```python
from build123d import *

# Parameters (mm, degrees)
SKETCH_1_W             = 35
SKETCH_1_H             = 70
SKETCH_1_R             = 2.6
EXTRUDE_528_DEPTH      = 3
SKETCH_2_R             = 2.1
CUT_EXTRUDE_M4_DEPTH   = 3
SKETCH_3_R             = 2.6
EXTRUDE_990_DEPTH      = 3
SKETCH_4_R             = 2.1
CUT_EXTRUDE_1335_DEPTH = 4
SKETCH_5_W             = 49
SKETCH_5_H             = 70
EXTRA_DEPTH            = 3
SKETCH_6_R             = 2.1
CUT_EXTRUDE_2079_DEPTH = 10
SKETCH_7_R             = 2.1
ETRA_DEPTH             = 10
SKETCH_10_R            = 1.6
SKETCH_10_R_2          = 3.5
CUT_EXTRUDE_3705_DEPTH = 4
FILLET_5_0_R           = 5
SKETCH_12_R            = 2.1
EXTRUDE_1_DEPTH        = 3
SKETCH_13_R            = 1.5
CUT_EXTRUDE_1_DEPTH    = 4
SKETCH_14_R            = 1.5
EXTRUDE_2_DEPTH        = 3
SKETCH_15_R            = 2.5
CUT_EXTRUDE_2_DEPTH    = 4
SKETCH_16_R            = 2.6
EXTRUDE_3_DEPTH        = 3
SKETCH_18_R            = 2.5
CUT_EXTRUDE_3_DEPTH    = 3
SKETCH_19_R            = 2.180798689
SKETCH_19_R_2          = 1.661770768
EXTRUDE_4_DEPTH        = 3
SKETCH_20_R            = 2.5
CUT_EXTRUDE_4_DEPTH    = 4
SKETCH_21_R            = 1.5
SKETCH_21_R_2          = 2.5
SKETCH_21_R_3          = 2.1
EXTRUDE_5_DEPTH        = 3
SKETCH_22_R            = 1.5
CUT_EXTRUDE_5_DEPTH    = 4
SKETCH_23_R            = 1.5
EXTRUDE_6_DEPTH        = 3
SKETCH_24_R            = 1.2
CUT_EXTRUDE_8_DEPTH    = 4
SKETCH_26_R            = 1.5
CUT_EXTRUDE_10_DEPTH   = 4
SKETCH_27_R            = 1.2
SKETCH_27_R_2          = 1.228912634
EXTRUDE_7_DEPTH        = 3
SKETCH_28_R            = 2.5
EXTRUDE_8_DEPTH        = 3
SKETCH_29_R            = 1.2
CUT_EXTRUDE_11_DEPTH   = 4
SKETCH_30_R            = 1.5
EXTRUDE_9_DEPTH        = 3
SKETCH_31_R            = 2.5
CUT_EXTRUDE_12_DEPTH   = 4
SKETCH_32_R            = 2.622023652
SKETCH_32_R_2          = 2.1
EXTRUDE_10_DEPTH       = 3
SKETCH_34_R            = 2.5
EXTRUDE_11_DEPTH       = 3
SKETCH_35_R            = 1.2
CUT_EXTRUDE_13_DEPTH   = 4
SKETCH_37_R            = 1.6
SKETCH_37_R_2          = 2.6
CUT_EXTRUDE_14_DEPTH   = 4


with BuildPart() as part:
    # 草图1 → Extrude 528 (new body)
    with BuildSketch(Plane(origin=(0, 0, 0), x_dir=(1, 0, 0), z_dir=(0, 1, 0))):
        Rectangle(SKETCH_1_W, SKETCH_1_H)
        with Locations((-7.5, 22.5)):
            Circle(SKETCH_1_R, mode=Mode.SUBTRACT)
        with Locations((-7.5, 0)):
            Circle(SKETCH_1_R, mode=Mode.SUBTRACT)
        with Locations((-7.5, -22.5)):
            Circle(SKETCH_1_R, mode=Mode.SUBTRACT)
        with Locations((-7.5, 10)):
            Circle(SKETCH_1_R, mode=Mode.SUBTRACT)
        with Locations((-7.5, -10)):
            Circle(SKETCH_1_R, mode=Mode.SUBTRACT)
    extrude(amount=EXTRUDE_528_DEPTH)

    # 草图2 → M4铝柱 (cut)
    with BuildSketch(Plane(origin=(0, 3, 0), x_dir=(1, 0, 0), z_dir=(0, 1, 0))):
        with Locations((10, 0)):
            Circle(SKETCH_2_R)
    extrude(amount=-CUT_EXTRUDE_M4_DEPTH, mode=Mode.SUBTRACT)

    # 草图3 → Extrude 990 (add, through all)
    with BuildSketch(Plane(origin=(0, 3, 0), x_dir=(1, 0, 0), z_dir=(0, 1, 0))):
        with Locations((-7.5, -10)):
            Circle(SKETCH_3_R)
        with Locations((-7.5, 10)):
            Circle(SKETCH_3_R)
    extrude(amount=-EXTRUDE_990_DEPTH)

    # 草图4 → Cut-Extrude 1335 (cut, through all)
    with BuildSketch(Plane(origin=(0, 3, 0), x_dir=(1, 0, 0), z_dir=(0, 1, 0))):
        with Locations((10, 22.5)):
            Circle(SKETCH_4_R)
        with Locations((10, -22.5)):
            Circle(SKETCH_4_R)
    extrude(amount=-CUT_EXTRUDE_1335_DEPTH, mode=Mode.SUBTRACT)

    # 草图5 → EXTRA (add, through all)
    with BuildSketch(Plane(origin=(0, 3, 0), x_dir=(1, 0, 0), z_dir=(0, 1, 0))):
        with Locations((-42, 0)):
            Rectangle(SKETCH_5_W, SKETCH_5_H)
    extrude(amount=-EXTRA_DEPTH)

    # 草图6 → Cut-Extrude 2079 (cut)
    with BuildSketch(Plane(origin=(0, 3, 0), x_dir=(1, 0, 0), z_dir=(0, 1, 0))):
        with Locations((-44.5, 0)):
            Circle(SKETCH_6_R)
        with Locations((-36.5, 0)):
            Circle(SKETCH_6_R)
    extrude(amount=-CUT_EXTRUDE_2079_DEPTH, mode=Mode.SUBTRACT)

    # 草图7 → ETRA铝柱 (cut)
    with BuildSketch(Plane(origin=(0, 3, 0), x_dir=(1, 0, 0), z_dir=(0, 1, 0))):
        with Locations((-56.5, 17.5)):
            Circle(SKETCH_7_R)
        with Locations((-56.5, -17.5)):
            Circle(SKETCH_7_R)
    extrude(amount=-ETRA_DEPTH, mode=Mode.SUBTRACT)

    # 草图10 → Cut-Extrude 3705 (cut, through all)
    with BuildSketch(Plane.XZ):
        with Locations((-43.5, -21.25)):
            Circle(SKETCH_10_R)
        with Locations((-21.5, -31.75)):
            Circle(SKETCH_10_R)
        with Locations((-43.5, -31.75)):
            Circle(SKETCH_10_R)
        with Locations((-43.5, 21.25)):
            Circle(SKETCH_10_R)
        with Locations((-21.5, 31.75)):
            Circle(SKETCH_10_R)
        with Locations((-43.5, 31.75)):
            Circle(SKETCH_10_R)
        with Locations((-21.5, 21.25)):
            Circle(SKETCH_10_R_2)
        with Locations((-21.5, -21.25)):
            Circle(SKETCH_10_R_2)
    extrude(amount=-CUT_EXTRUDE_3705_DEPTH, mode=Mode.SUBTRACT)

    # 圆角5.0
    fillet_5_0_edges = [part.edges().sort_by_distance(p)[0] for p in [
        (-66.5, 1.5, 35),
        (-66.5, 1.5, -35),
        (17.5, 1.5, 35),
        (17.5, 1.5, -35),
    ]]
    fillet(fillet_5_0_edges, radius=FILLET_5_0_R)

    # 草图12 → 凸台-拉伸1 (add)
    with BuildSketch(Plane(origin=(0, 3, 0), x_dir=(1, 0, 0), z_dir=(0, 1, 0))):
        with Locations((-36.5, 0)):
            Circle(SKETCH_12_R)
        with Locations((-44.5, 0)):
            Circle(SKETCH_12_R)
    extrude(amount=-EXTRUDE_1_DEPTH)

    # 草图13 → 切除-拉伸1 (cut, through all)
    with BuildSketch(Plane(origin=(0, 3, 0), x_dir=(1, 0, 0), z_dir=(0, 1, 0))):
        with Locations((-52.499999555, 1.426e-06)):
            Circle(SKETCH_13_R)
        with Locations((-28.499999555, 1.44e-06)):
            Circle(SKETCH_13_R)
    extrude(amount=-CUT_EXTRUDE_1_DEPTH, mode=Mode.SUBTRACT)

    # 草图14 → 凸台-拉伸2 (add)
    with BuildSketch(Plane(origin=(0, 3, 0), x_dir=(1, 0, 0), z_dir=(0, 1, 0))):
        with Locations((-28.499999555, 1.44e-06)):
            Circle(SKETCH_14_R)
    extrude(amount=-EXTRUDE_2_DEPTH)

    # 草图15 → 切除-拉伸2 (cut, through all)
    with BuildSketch(Plane(origin=(0, 3, 0), x_dir=(1, 0, 0), z_dir=(0, 1, 0))):
        with Locations((-23.393651392, 12.166497951)):
            Circle(SKETCH_15_R)
        with Locations((-23.393651594, -11.919830539)):
            Circle(SKETCH_15_R)
    extrude(amount=-CUT_EXTRUDE_2_DEPTH, mode=Mode.SUBTRACT)

    # 草图16 → 凸台-拉伸3 (add)
    with BuildSketch(Plane(origin=(0, 3, 0), x_dir=(1, 0, 0), z_dir=(0, 1, 0))):
        with Locations((-7.5, 22.5)):
            Circle(SKETCH_16_R)
        with Locations((-7.5, 0)):
            Circle(SKETCH_16_R)
        with Locations((-7.5, -22.5)):
            Circle(SKETCH_16_R)
    extrude(amount=-EXTRUDE_3_DEPTH)

    # 草图18 → 切除-拉伸3 (cut)
    with BuildSketch(Plane.XZ):
        with Locations((-3.558761246, 0)):
            Circle(SKETCH_18_R)
        with Locations((-3.558761246, 22.202338419)):
            Circle(SKETCH_18_R)
        with Locations((-3.558761246, -23.518793957)):
            Circle(SKETCH_18_R)
    extrude(amount=-CUT_EXTRUDE_3_DEPTH, mode=Mode.SUBTRACT)

    # 草图19 → 凸台-拉伸4 (add)
    with BuildSketch(Plane.XZ):
        with Locations((-43.5, 21.25)):
            Circle(SKETCH_19_R)
        with Locations((-43.5, 31.75)):
            Circle(SKETCH_19_R_2)
    extrude(amount=-EXTRUDE_4_DEPTH)

    # 草图20 → 切除-拉伸4 (cut, through all)
    with BuildSketch(Plane(origin=(0, 3, 0), x_dir=(1, 0, 0), z_dir=(0, 1, 0))):
        with Locations((-40.5, 1.551947464)):
            Circle(SKETCH_20_R)
        with Locations((-40.5, -18.448052536)):
            Circle(SKETCH_20_R)
    extrude(amount=-CUT_EXTRUDE_4_DEPTH, mode=Mode.SUBTRACT)

    # 草图21 → 凸台-拉伸5 (add)
    with BuildSketch(Plane(origin=(0, 3, 0), x_dir=(1, 0, 0), z_dir=(0, 1, 0))):
        with Locations((-52.499999555, 1.426e-06)):
            Circle(SKETCH_21_R)
        with Locations((-40.5, 1.551947464)):
            Circle(SKETCH_21_R_2)
        with Locations((-3.558761246, 0)):
            Circle(SKETCH_21_R_2)
        with Locations((10, 0)):
            Circle(SKETCH_21_R_3)
    extrude(amount=-EXTRUDE_5_DEPTH)

    # 草图22 → 切除-拉伸5 (cut, through all)
    with BuildSketch(Plane(origin=(0, 3, 0), x_dir=(1, 0, 0), z_dir=(0, 1, 0))):
        with Locations((-52.5, 0)):
            Circle(SKETCH_22_R)
        with Locations((-28.5, 0)):
            Circle(SKETCH_22_R)
    extrude(amount=-CUT_EXTRUDE_5_DEPTH, mode=Mode.SUBTRACT)

    # 草图23 → 凸台-拉伸6 (add)
    with BuildSketch(Plane(origin=(0, 3, 0), x_dir=(1, 0, 0), z_dir=(0, 1, 0))):
        with Locations((-52.5, 0)):
            Circle(SKETCH_23_R)
        with Locations((-28.5, 0)):
            Circle(SKETCH_23_R)
    extrude(amount=-EXTRUDE_6_DEPTH)

    # 草图24 → 切除-拉伸8 (cut, through all)
    with BuildSketch(Plane(origin=(0, 3, 0), x_dir=(1, 0, 0), z_dir=(0, 1, 0))):
        with Locations((-45.5, -0.064794531)):
            Circle(SKETCH_24_R)
        with Locations((-25.5, -0.064794531)):
            Circle(SKETCH_24_R)
    extrude(amount=-CUT_EXTRUDE_8_DEPTH, mode=Mode.SUBTRACT)

    # 草图26 → 切除-拉伸10 (cut, through all)
    with BuildSketch(Plane.XZ):
        with Locations((-52.5, 0)):
            Circle(SKETCH_26_R)
        with Locations((-28.5, 0)):
            Circle(SKETCH_26_R)
    extrude(amount=-CUT_EXTRUDE_10_DEPTH, mode=Mode.SUBTRACT)

    # 草图27 → 凸台-拉伸7 (add)
    with BuildSketch(Plane(origin=(0, 0, 0), x_dir=(-1, 0, 0), z_dir=(0, -1, 0))):
        with Locations((25.5, -0.064794531)):
            Circle(SKETCH_27_R)
        with Locations((45.5, -0.064794531)):
            Circle(SKETCH_27_R_2)
    extrude(amount=-EXTRUDE_7_DEPTH)

    # 草图28 → 凸台-拉伸8 (add)
    with BuildSketch(Plane(origin=(0, 3, 0), x_dir=(1, 0, 0), z_dir=(0, 1, 0))):
        with Locations((-3.558761246, -22.202338419)):
            Circle(SKETCH_28_R)
        with Locations((-3.558761246, 23.518793957)):
            Circle(SKETCH_28_R)
    extrude(amount=-EXTRUDE_8_DEPTH)

    # 草图29 → 切除-拉伸11 (cut, through all)
    with BuildSketch(Plane(origin=(0, 3, 0), x_dir=(1, 0, 0), z_dir=(0, 1, 0))):
        with Locations((-25.5, -0.064794531)):
            Circle(SKETCH_29_R)
        with Locations((-45.5, -0.064794531)):
            Circle(SKETCH_29_R)
    extrude(amount=-CUT_EXTRUDE_11_DEPTH, mode=Mode.SUBTRACT)

    # 草图30 → 凸台-拉伸9 (add)
    with BuildSketch(Plane(origin=(0, 3, 0), x_dir=(1, 0, 0), z_dir=(0, 1, 0))):
        with Locations((-28.5, 0)):
            Circle(SKETCH_30_R)
        with Locations((-52.5, 0)):
            Circle(SKETCH_30_R)
    extrude(amount=-EXTRUDE_9_DEPTH)

    # 草图31 → 切除-拉伸12 (cut, through all)
    with BuildSketch(Plane.XZ):
        with Locations((-5, 25.879055361)):
            Circle(SKETCH_31_R)
        with Locations((-5, -25.879055361)):
            Circle(SKETCH_31_R)
    extrude(amount=-CUT_EXTRUDE_12_DEPTH, mode=Mode.SUBTRACT)

    # 草图32 → 凸台-拉伸10 (add)
    with BuildSketch(Plane(origin=(0, 3, 0), x_dir=(1, 0, 0), z_dir=(0, 1, 0))):
        with Locations((10, -22.5)):
            Circle(SKETCH_32_R)
        with Locations((10, 22.5)):
            Circle(SKETCH_32_R_2)
    extrude(amount=-EXTRUDE_10_DEPTH)

    # 草图34 → 凸台-拉伸11 (add)
    with BuildSketch(Plane(origin=(0, 3, 0), x_dir=(1, 0, 0), z_dir=(0, 1, 0))):
        with Locations((-23.393651392, 12.166497951)):
            Circle(SKETCH_34_R)
    extrude(amount=-EXTRUDE_11_DEPTH)

    # 草图35 → 切除-拉伸13 (cut, through all)
    with BuildSketch(Plane(origin=(0, 3, 0), x_dir=(1, 0, 0), z_dir=(0, 1, 0))):
        with Locations((-5.06603585, 9.935205469)):
            Circle(SKETCH_35_R)
        with Locations((-25.06603585, 9.935205469)):
            Circle(SKETCH_35_R)
    extrude(amount=-CUT_EXTRUDE_13_DEPTH, mode=Mode.SUBTRACT)

    # 草图37 → 切除-拉伸14 (cut, through all)
    with BuildSketch(Plane(origin=(0, 3, 0), x_dir=(1, 0, 0), z_dir=(0, 1, 0))):
        with Locations((-45.5, -0.064794531)):
            Circle(SKETCH_37_R)
        with Locations((-25.5, -0.064794531)):
            Circle(SKETCH_37_R)
        with Locations((-25.06603585, 9.935205469)):
            Circle(SKETCH_37_R)
        with Locations((-5.06603585, 9.935205469)):
            Circle(SKETCH_37_R)
        with Locations((-5, 25.879055361)):
            Circle(SKETCH_37_R_2)
        with Locations((-5, -25.879055361)):
            Circle(SKETCH_37_R_2)
        with Locations((-56.5, 17.5)):
            Circle(SKETCH_37_R_2)
        with Locations((-56.5, -17.5)):
            Circle(SKETCH_37_R_2)
    extrude(amount=-CUT_EXTRUDE_14_DEPTH, mode=Mode.SUBTRACT)


solid = part.part
```
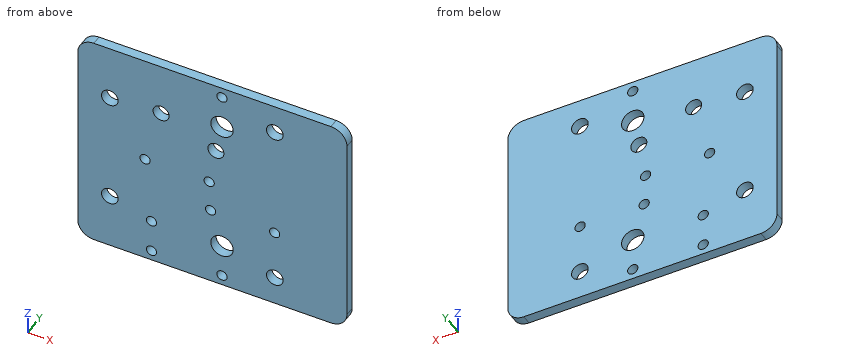
Could you check a few things on this model? Use its own coordinates, in mm. Round coordinates to 2 decimals unless told otherwise and drop trailing zeros. Loops run counter-clockwise (first coordinate to the right, second up) from the corner with the lowest first, then second, coordinate; pieces in that order, holes last. Notation, with made-up numbers: (-31, 89) -> (-9, 89) arc R13 ccw to (-9, 94) -> close; hole circle Ø10 at (9.25, 59). An arc over 180 degrees is marked (long way). One line per question, with ' | ' between items.
(1) If we section it at B-B on x = -56.5: List the corners of the cut face in (y, z) for me, and give its area (3 significant figures).
Model answer:
outline: (0, -35) -> (3, -35) -> (3, -20.1) -> (0, -20.1) -> close; (0, -14.9) -> (3, -14.9) -> (3, 14.9) -> (0, 14.9) -> close; (0, 20.1) -> (3, 20.1) -> (3, 35) -> (0, 35) -> close | area: 179 mm^2
(2) If we section it at C-C on y = 1.2: Count the separate pieces of the cut face and the enclosed holes in it, and give its area (3 significant figures).
Model answer:
separate pieces: 1 | enclosed holes: 16 | area: 5,590 mm^2
(3) For pin 1 Ø3 at (x, z) = (-43.5, -21.25) entering from -Y, with a flat end and sliding along its axis, tell me the tip position at first contact or that it passes through.
Model answer:
pin 1: passes through
(4) If I drill on probe 1 along Z at (x, y) = (-43.5, 2.45); probe 2 along X at (y, z) = (2.3, -19); probe 3 along Z at (x, y) = (-21.5, 0.95), over which ranges is the centre line in solid material (lowest first)?
Model answer:
probe 1: z = -35 to -33.35, -30.15 to -22.85, -19.65 to 35 | probe 2: x = -66.5 to -58.62, -54.38 to -24.18, -18.82 to 17.5 | probe 3: z = -35 to -33.35, -30.15 to -24.75, -17.75 to 10.29, 13.55 to 17.75, 24.75 to 30.15, 33.35 to 35
(5) If we section it at D-D on x = -41: List the corners of the cut face in (y, z) for me.
Model answer:
outline: (0, -35) -> (3, -35) -> (3, 16) -> (0, 16) -> close; (0, 20.9) -> (3, 20.9) -> (3, 35) -> (0, 35) -> close
(6) If we section it at A-A on z = -21.25: List the corners of the cut face in (x, y) for me, and give its area (3 significant figures).
Model answer:
outline: (-66.5, 0) -> (-45.1, 0) -> (-45.1, 3) -> (-66.5, 3) -> close; (-41.9, 0) -> (-25, 0) -> (-25, 3) -> (-41.9, 3) -> close; (-18, 0) -> (17.5, 0) -> (17.5, 3) -> (-18, 3) -> close | area: 221 mm^2
